```python
from build123d import *

# Parameters (mm, degrees)
F1_DEPTH = 6.35
F2_DEPTH = 6.35
F3_DEPTH = 6.35
F0_R     = 1.905
F4_DEPTH = 6.35


with BuildPart() as f1:
    # F0 (on Front) → F1 (new body)
    with BuildSketch(Plane.XZ):
        with BuildLine():
            Line((3.81, -117.7925), (3.81, -15.737883))
            ThreePointArc((3.81, -15.737883), (0, -16.1925), (-3.81, -15.737883))
            Line((-3.81, -15.737883), (-3.81, -117.7925))
            Line((-3.81, -117.7925), (3.81, -117.7925))
        make_face()
    extrude(amount=F1_DEPTH)



with BuildPart() as f2:
    # F0 (on Front) → F2 (new body)
    with BuildSketch(Plane.XZ):
        with BuildLine():
            Line((3.81, -12.447458), (3.81, -15.737883))
            ThreePointArc((3.81, -15.737883), (12.725771, -10.012583), (16.1925, 0))
            ThreePointArc((16.1925, 0), (12.725771, 10.012583), (3.81, 15.737883))
            Line((3.81, 15.737883), (3.81, 12.447458))
            ThreePointArc((3.81, 12.447458), (10.465467, 7.741403), (13.0175, 0))
            ThreePointArc((13.0175, 0), (10.465467, -7.741403), (3.81, -12.447458))
        make_face()
        with BuildLine():
            ThreePointArc((-3.81, 15.737883), (-16.1925, 0), (-3.81, -15.737883))
            Line((-3.81, -15.737883), (-3.81, -12.447458))
            ThreePointArc((-3.81, -12.447458), (-13.0175, 0), (-3.81, 12.447458))
            Line((-3.81, 12.447458), (-3.81, 15.737883))
        make_face()
    extrude(amount=F2_DEPTH)


with BuildPart() as f1_1:
    add(f1.part)

    add(f2.part)  # F3 merges F2
    # F0 (on Front) → F3 (join, symmetric)
    with BuildSketch(Plane.XZ):
        with BuildLine():
            Line((3.81, 12.447458), (3.81, 15.737883))
            ThreePointArc((3.81, 15.737883), (0, 16.1925), (-3.81, 15.737883))
            Line((-3.81, 15.737883), (-3.81, 12.447458))
            ThreePointArc((-3.81, 12.447458), (0, 13.0175), (3.81, 12.447458))
        make_face()
        with BuildLine():
            ThreePointArc((-3.81, -15.737883), (0, -16.1925), (3.81, -15.737883))
            Line((3.81, -15.737883), (3.81, -12.447458))
            ThreePointArc((3.81, -12.447458), (0, -13.0175), (-3.81, -12.447458))
            Line((-3.81, -12.447458), (-3.81, -15.737883))
        make_face()
    extrude(amount=F3_DEPTH, both=True)

    # F0 (on Front) → F4 (join)
    with BuildSketch(Plane.XZ):
        with BuildLine():
            ThreePointArc((-3.81, -12.447458), (0, -13.0175), (3.81, -12.447458))
            Line((3.81, -12.447458), (3.81, 12.447458))
            ThreePointArc((3.81, 12.447458), (0, 13.0175), (-3.81, 12.447458))
            Line((-3.81, 12.447458), (-3.81, -12.447458))
        make_face()
        Circle(F0_R, mode=Mode.SUBTRACT)
    extrude(amount=-F4_DEPTH)


solid = f1_1.part
```
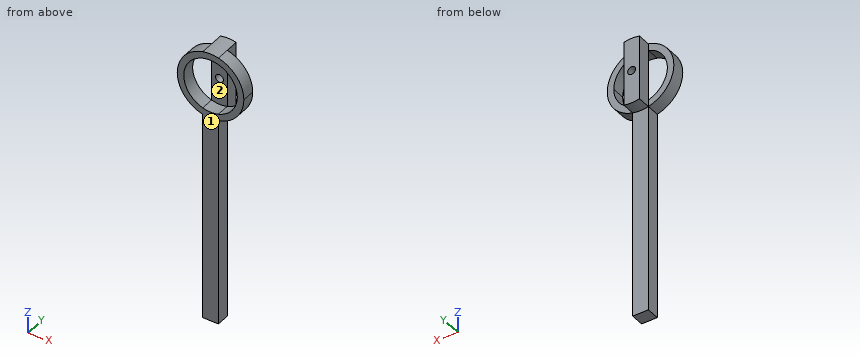
Geometry: final body of the model. Coordinates: model frame, mm. Face numbers are marked on the shaded views. Round coordinates to 2 decimals unless told otherwise and drop trailing zeros. Write each loop counter-clockwise with the first axis right and the second up, starting at its lowest first coordinate (ties: lowest second). Pieces come first, ordered by that corner, then holes.
Item 1: Section query C-C (z = -8). Return loops of the section in (x, y).
Item 2: Mould query, pull axis Z, two halves, no side actions, for the marked faces 1 and 2. Classes: +Z half, -Z half, draft (parallel to the pull), parting line (faces both ways), or undercut.
Item 3: Section query A-A (y = -4.25). Return loops of the section in (x, z) (1 decimal).
Item 4: Material intervals for L1, parallel to Z at x = -10, y = -4; L2, parallel to Y at x = 3.5, z = -40; L3, parallel to X at y = -1.75, z = -42, sorted ascending.
Item 5: Pin query (flat end, axial travel): P1, Ø1, axis at x = 7, y = -4.5, coming from the -Z side; P2, Ø3.5, axis at x = 0, z = 0, coming from the -Y side; P3, Ø1.9, axis at y = -2.5, z = -85.5, coming from the +X side; P4, Ø1, axis at x = 3, z = -11.5, coming from the -Y side. Return the tip coordinate at first contact, or that it passes through.
Item 6: Section query D-D (x = 6). Return loops of the section in (y, z), plus the area to 3 significant figures.
Completed:
1. outline: (-14.08, -6.35) - (-10.27, -6.35) - (-10.27, 0) - (-14.08, 0) - close; (-3.81, 0) - (3.81, 0) - (3.81, 6.35) - (-3.81, 6.35) - close; (10.27, -6.35) - (14.08, -6.35) - (14.08, 0) - (10.27, 0) - close
2. face 1: draft
2. face 2: undercut
3. outline: (-3.8, -117.8) - (3.8, -117.8) - (3.8, -15.7) arc R16.2 ccw to (16.2, 0) arc R16.2 ccw to (3.8, 15.7) arc R16.2 ccw to (-3.8, 15.7) arc R16.2 ccw to (-3.8, -15.7) - close; hole (-3.8, -12.4) arc R13 ccw to (3.8, -12.4) arc R13 ccw to (13, 0) arc R13 ccw to (3.8, 12.4) arc R13 ccw to (-3.8, 12.4) arc R13 ccw to start
4. L1: z = -12.74 to -8.33, 8.33 to 12.74
4. L2: y = -6.35 to 0
4. L3: x = -3.81 to 3.81
5. P1: stops at z = -14.83
5. P2: passes through
5. P3: stops at x = 3.81
5. P4: stops at y = 0
6. outline: (-6.35, -15.04) - (0, -15.04) - (0, -11.55) - (-6.35, -11.55) - close; (-6.35, 11.55) - (0, 11.55) - (0, 15.04) - (-6.35, 15.04) - close
6. area: 44.3 mm2
